Input: dimensioned drawing with shaded views. Units: mm. Origin: part minimum x, y, z. A direction names the side the tool comes from. Coordinates: 2 decimals unless noted, no trailing zeros. Loops run counter-clockwise (first coordinate to the right, second up) from the corner with the lowest first, then second, coordinate; pieces in that order, holes last. Notation, with made-up numbers: (9.5, 72) - (41.5, 72) arc R25 cw to (41.5, 104) - close; hole circle Ø9 at (-4.75, 47.5). An arc over 180 degrees is marked (long way). Put each result on its own line as item: value. Start each with the question number.
1) Material intervals for line 1 along Y through (x, z) = (61.5, 6.5); line 2 along X through (y, z) = (34, 25.5) (1 decimal); line 3 along Y through (x, z) = (3, 24.5), sorted ascending. Write a range as from..to.
2) Contact query for flat-ended pins moving along their axis: pin 1 Ø3 at (x, z) = (30.5, 18) entering from +Y; pin 2 Ø1.8 at (x, z) = (31, 23) entering from -Y; pin 3 Ø5 at (y, z) = (28.5, 14.5) entering from -X. Output: stop coordinate, or through.
3) Draft query along X for the marked faces 1, 2, 3 and 4. Return one class per face: +X half, -X half, draft (parallel to the pull), parting line (faces both ways), or undercut.
4) Section D-D on z = 20. Output: boundary loops of the cut face in (x, y).
5) Section B-B on y = 14.5. Output: boundary loops of the cut face in (x, z), and give its area (3 significant figures).
6) Section A-A on z = 29.5. Output: boundary loops of the cut face in (x, y), and give its area (3 significant figures).
7) Section C-C on y = 42. Output: boundary loops of the cut face in (x, z), and give its area (3 significant figures).
8) Reachability of the marked faces 5, 6, 7, 8 and 9 from +Z, -Z, +X, -X, +Y, -Y: full face, straight path, thin tool, end or side. Return the list, or none.
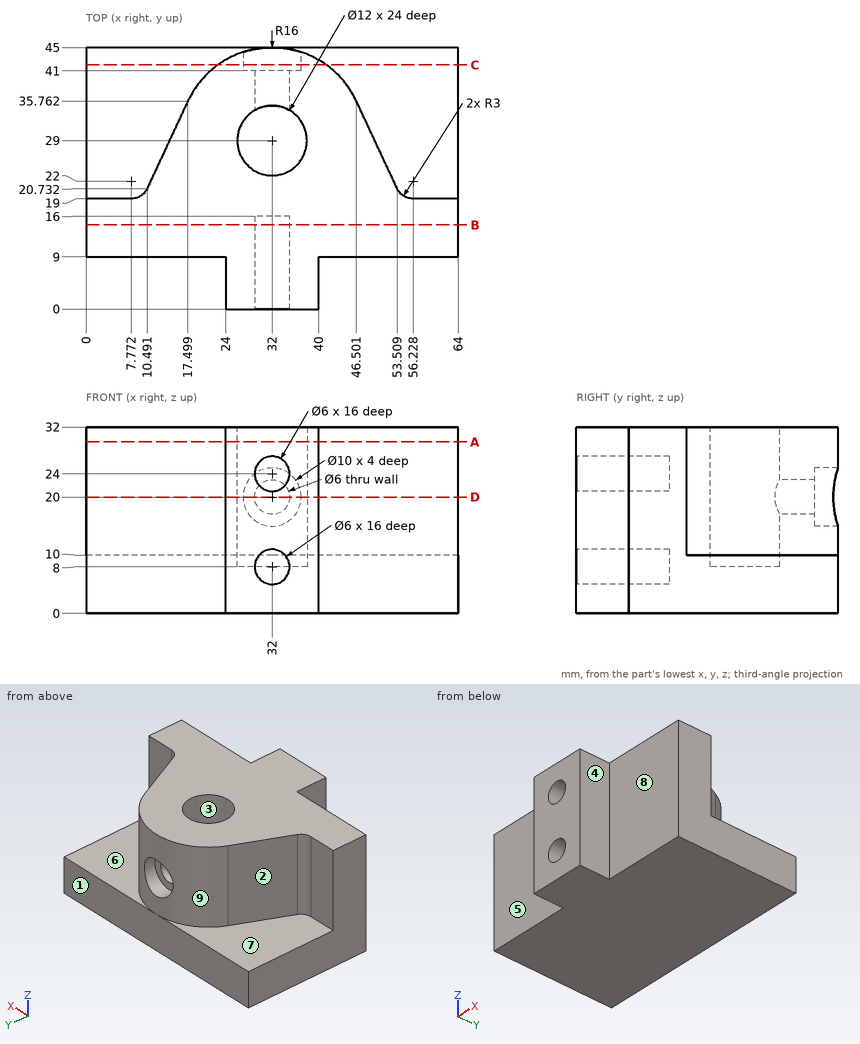
Answer block:
1. line 1: y = 9..45
1. line 2: x = 16.7..28.7, 35.3..47.3
1. line 3: y = 9..19
2. pin 1: stops at y = 41
2. pin 2: stops at y = 16
2. pin 3: stops at x = 12.95
3. face 1: draft
3. face 2: -X half
3. face 3: undercut
3. face 4: +X half
4. outline: (0, 9) - (24, 9) - (24, 0) - (40, 0) - (40, 9) - (64, 9) - (64, 19) - (56.23, 19) arc R3 cw to (53.51, 20.73) - (46.5, 35.76) arc R16 ccw to (37, 44.2) - (37, 41) - (35, 41) - (35, 34.2) arc R6 cw (long way) to (29, 34.2) - (29, 41) - (27, 41) - (27, 44.2) arc R16 ccw to (17.5, 35.76) - (10.49, 20.73) arc R3 cw to (7.77, 19) - (0, 19) - close
5. outline: (0, 0) - (64, 0) - (64, 32) - (0, 32) - close; hole circle Ø6 at (32, 8); hole circle Ø6 at (32, 24)
5. area: 1,990 mm²
6. outline: (0, 9) - (24, 9) - (24, 0) - (40, 0) - (40, 9) - (64, 9) - (64, 19) - (56.23, 19) arc R3 cw to (53.51, 20.73) - (46.5, 35.76) arc R16 ccw to (17.5, 35.76) - (10.49, 20.73) arc R3 cw to (7.77, 19) - (0, 19) - close; hole circle Ø12 at (32, 29)
6. area: 1,480 mm²
7. outline: (0, 0) - (64, 0) - (64, 10) - (41.33, 10) - (41.33, 32) - (22.67, 32) - (22.67, 10) - (0, 10) - close; hole circle Ø10 at (32, 20)
7. area: 972 mm²
8. face 5: +Z, -Z, -X, -Y
8. face 6: +Z, +X, +Y
8. face 7: +Z, -X, +Y
8. face 8: +Z, -Z, +X, -Y
8. face 9: +Z, +Y
